```python
from build123d import *

# Parameters (mm, degrees)
SKETCH_1_R          = 3.5
EXTRUDE_1_DEPTH     = 90
CUT_EXTRUDE_1_DEPTH = 2
SKETCH_3_R          = 3.5
SKETCH_3_R_2        = 2.1
CUT_EXTRUDE_3_DEPTH = 2
SKETCH_4_R          = 0.548210007
EXTRUDE_2_DEPTH     = 2
SKETCH_5_R          = 1.45
CUT_EXTRUDE_5_DEPTH = 10


with BuildPart() as part:
    # 草图1 → 凸台-拉伸1 (new body)
    with BuildSketch(Plane(origin=(0, 0, 0), x_dir=(1, 0, 0), z_dir=(0, 1, 0))):
        with Locations(Location((0, 0, 0), (0, 0, 90))):
            Circle(SKETCH_1_R)
    extrude(amount=EXTRUDE_1_DEPTH)

    # 草图2 → 切除-拉伸1 (cut)
    with BuildSketch(Plane.XZ):
        with BuildLine():
            Line((0, 3.5), (0, 2.1))
            ThreePointArc((0, 2.1), (1.698935688, 1.23434903), (1.997218684, -0.648935688))
            Line((1.997218684, -0.648935688), (3.328697807, -1.08155948))
            ThreePointArc((3.328697807, -1.08155948), (3.456909192, -0.547520628), (3.5, 0))
            ThreePointArc((3.5, 0), (2.474873734, 2.474873734), (0, 3.5))
        make_face()
        with BuildLine():
            ThreePointArc((0, -2.1), (-1.698935688, -1.23434903), (-1.997218684, 0.648935688))
            Line((-1.997218684, 0.648935688), (-3.328697807, 1.08155948))
            ThreePointArc((-3.328697807, 1.08155948), (-2.83155948, -2.057248383), (0, -3.5))
            Line((0, -3.5), (0, -2.1))
        make_face()
    extrude(amount=-CUT_EXTRUDE_1_DEPTH, mode=Mode.SUBTRACT)

    # 草图3 → 切除-拉伸3 (cut)
    with BuildSketch(Plane.XZ.offset(-2)):
        with Locations(Location((0, 0, 0), (0, 0, 270))):
            Circle(SKETCH_3_R)
        with Locations(Location((0, 0, 0), (0, 0, 270))):
            Circle(SKETCH_3_R_2, mode=Mode.SUBTRACT)
    extrude(amount=-CUT_EXTRUDE_3_DEPTH, mode=Mode.SUBTRACT)

    # 草图4 → 凸台-拉伸2 (add)
    with BuildSketch(Plane(origin=(0, 2, 0), x_dir=(1, 0, 0), z_dir=(0, 1, 0))):
        with Locations((-1.025992333, -1.768146991)):
            Circle(SKETCH_4_R)
        with Locations((1.025992333, 1.768146991)):
            Circle(SKETCH_4_R)
    extrude(amount=EXTRUDE_2_DEPTH)

    # 草图5 → 切除-拉伸5 (cut)
    with BuildSketch(Plane(origin=(0, 90, 0), x_dir=(1, 0, 0), z_dir=(0, 1, 0))):
        with Locations(Location((0, 0, 0), (0, 0, 270))):
            Circle(SKETCH_5_R)
    extrude(amount=-CUT_EXTRUDE_5_DEPTH, mode=Mode.SUBTRACT)

    # 草图6 → 切除-旋转2 (revolve, cut)
    with BuildSketch(Plane.XY, mode=Mode.PRIVATE) as cut_revolve_2_sk:
        with BuildLine():
            Line((3.5, 90), (3.5, 89.7))
            add(Edge.make_bspline(
                [(3.5, 89.7), (2.810594715, 89.888843462), (2.108922974, 89.988601578), (1.395404454, 90)],
                knots=[0, 0, 0, 0, 0.917895011, 0.917895011, 0.917895011, 0.917895011], degree=3))
            Line((1.395404454, 90), (3.5, 90))
        make_face()
    revolve(cut_revolve_2_sk.sketch.rotate(Axis((0, 107.628853611, 0), (0, -1, 0)), 270), axis=Axis((0, 107.628853611, 0), (0, -1, 0)), mode=Mode.SUBTRACT)


solid = part.part
```
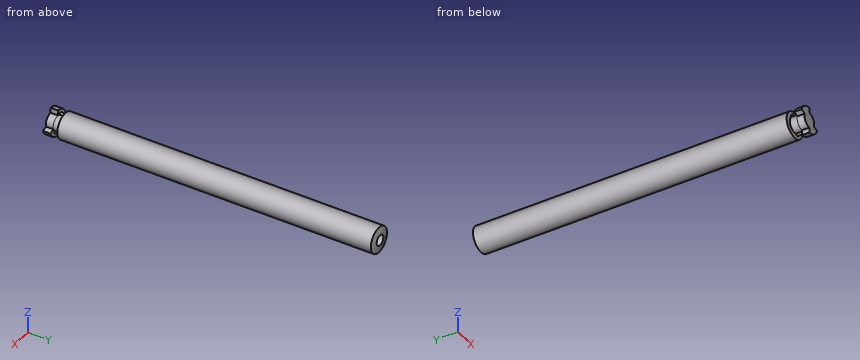
Check sheet for the modelled part. Datum: model origin and axes. Units: mm. Coordinates: 2 decimals unless noted, no trailing zeros. Write each loop counter-clockwise with the first axis right and the second up, starting at its lowest first coordinate (ties: lowest second). Pieces come first, ordered by that corner, then holes. Notation, with made-up numbers: (73, 47) -> (118, 47) arc R37 cw to (118, 84) -> close; hole circle Ø11 at (36, -10.75). An arc over 180 degrees is marked (long way). Use a Markdown table: item, result.
1. Scan lines: line 1 along X through (y, z) = (82.25, 0); line 2 along X through (y, z) = (29, -0.25); line 3 along Y through (x, z) = (2, -1.5). Record each from-to range of solid material in increasing order.
Reported:
| item | result |
|---|---|
| line 1 | x = -3.5 to -1.45, 1.45 to 3.5 |
| line 2 | x = -3.49 to 3.49 |
| line 3 | y = 0 to 2, 4 to 89.91 |
2. Go/stop test with flat-tipped pins: pin 1 Ø2 at (x, y) = (-2, 35) entering from +Z; pin 2 Ø3 at (x, z) = (0.5, 2.5) entering from +Y; pin 3 Ø1 at (y, z) = (66, -2) entering from -X; pin 4 Ø1.5 at (y, z) = (1.5, -2.5) entering from -X. Record where each tip stops, or that it passes through.
Reported:
| item | result |
|---|---|
| pin 1 | stops at z = 3.35 |
| pin 2 | stops at y = 90 |
| pin 3 | stops at x = -3.16 |
| pin 4 | stops at x = -1.16 |
3. Sectioned sample at A-A (y = 69.5). Enter the section's corners in (x, z).
Reported:
| item | result |
|---|---|
| outline | circle Ø7 at (0, 0) |
